```python
from build123d import *

# Parameters (mm, degrees)
SKETCH1_R           = 1.7859375
BOSS_EXTRUDE1_DEPTH = 1.5875
FILLET1_R           = 3.571875


with BuildPart() as part:
    # Sketch1 → Boss-Extrude1 (new body)
    with BuildSketch(Plane.XY):
        with BuildLine():
            ThreePointArc((31.75, -12.7), (35.321875, -9.128125), (31.75, -5.55625))
            ThreePointArc((31.75, -5.55625), (37.30625, 0), (31.75, 5.55625))
            Line((31.75, 5.55625), (25.964019559, 5.55625))
            ThreePointArc((25.964019559, 5.55625), (23.279229109, 11.484009389), (20.594438658, 5.55625))
            Line((20.594438658, 5.55625), (11.155561342, 5.55625))
            ThreePointArc((11.155561342, 5.55625), (8.470770891, 11.484009389), (5.785980441, 5.55625))
            Line((5.785980441, 5.55625), (0, 5.55625))
            ThreePointArc((0, 5.55625), (-5.55625, 0), (0, -5.55625))
            ThreePointArc((0, -5.55625), (-3.571875, -9.128125), (0, -12.7))
            ThreePointArc((0, -12.7), (8.980256121, -8.980256121), (12.7, 0))
            Line((12.7, 0), (19.05, 0))
            ThreePointArc((19.05, 0), (22.769743879, -8.980256121), (31.75, -12.7))
        make_face()
        with BuildLine():
            ThreePointArc((0, -10.9140625), (-1.7859375, -9.128125), (0, -7.3421875))
            ThreePointArc((0, -7.3421875), (5.413228446, -4.960309977), (7.31424826, 0.639913805))
            ThreePointArc((7.31424826, 0.639913805), (8.937735019, 2.574709983), (10.872531197, 0.951223224))
            ThreePointArc((10.872531197, 0.951223224), (8.046690934, -7.37343375), (0, -10.9140625))
        make_face(mode=Mode.SUBTRACT)
        with BuildLine():
            ThreePointArc((24.43575174, 0.639913805), (26.336771554, -4.960309977), (31.75, -7.3421875))
            ThreePointArc((31.75, -7.3421875), (33.5359375, -9.128125), (31.75, -10.9140625))
            ThreePointArc((31.75, -10.9140625), (23.703309066, -7.37343375), (20.877468803, 0.951223224))
            ThreePointArc((20.877468803, 0.951223224), (22.812264981, 2.574709983), (24.43575174, 0.639913805))
        make_face(mode=Mode.SUBTRACT)
        Circle(SKETCH1_R, mode=Mode.SUBTRACT)
        with Locations((8.470770891, 7.912134389)):
            Circle(SKETCH1_R, mode=Mode.SUBTRACT)
        with Locations((31.75, 0)):
            Circle(SKETCH1_R, mode=Mode.SUBTRACT)
        with Locations((23.279229109, 7.912134389)):
            Circle(SKETCH1_R, mode=Mode.SUBTRACT)
    extrude(amount=BOSS_EXTRUDE1_DEPTH)

    # Fillet1
    fillet1_edges = [part.edges().sort_by_distance(p)[0] for p in [
        (31.75, -5.55625, 0.79375),
        (19.05, 0, 0.79375),
        (12.7, 0, 0.79375),
        (0, -5.55625, 0.79375),
        (20.594438658, 5.55625, 0.79375),
        (25.964019559, 5.55625, 0.79375),
        (5.785980441, 5.55625, 0.79375),
        (11.155561342, 5.55625, 0.79375),
    ]]
    fillet(fillet1_edges, radius=FILLET1_R - 0.0001)  # a hair under: the kernel refuses the full size


solid = part.part
```
Source: CAD feature listing. Evaluate the final solid. Frame: model axes, mm. A direction names the side the tool comes from. Coordinates: 2 decimals unless noted, no trailing zeros. Loops run counter-clockwise (first coordinate to the right, second up) from the corner with the lowest first, then second, coordinate; pieces in that order, holes last. Notation, with made-up numbers: M 8.5,-10 L 43.5,-10 A25 ccw 43.5,17 Z; hole C 30,-10 d9. An arc over 180 degrees is marked long. Put each result on its own line as item: value. Start each with the question number.
1) Ray query, L1, parallel to Y at x = 31.75, z = 0.3; L2, parallel to X at y = -4.5, z = 0.35; L3, parallel to X at y = -6.5, z = 0.3. Return the intervals inside material, ascending. Write a range as from..to.
2) Contact query for flat-ended pins moving along their axis: pin 1 Ø3 at (x, y) = (31.75, 0) entering from -Z; pin 2 Ø4 at (x, y) = (8.47, 7.91) entering from -Z. Output: stop coordinate, or through.
3) Cut plane A-A on y = -10.5. Return the cut outline in (x, z), then the cut area to 3 significant figures.
4) Cut plane D-D on z = 0.8. Give the number of separate pieces and of enclosed holes in the cut face, then the cut area to 3 significant figures.
5) Pull-direction query (Y, two-part tool) for faces 1 (the face through (16, 2, 0)), 2 (the face through (8.541, 11.483, 0.783)), 3 (the face through (23.789, -7.466, 0.783)), 4 (the face through (23.72, -9.84, 0.78)); classes: pulls with the +Y half, pulls with the -Y half, needs draft (parallel to the pull), parting line crosses it, or undercut.
6) Cut plane C-C on x = 24. Return the cut outline in (y, z), then the cut area to 3 significant figures.
7) Cut plane B-B on x = 6. Return the cut outline in (y, z), then the cut area to 3 significant figures.
8) Reachability of faces 5 (the face through (22.773, 2.578, 0.783)), 6 (the face through (18.13, -0.8, 0.8)), 7 (the face through (31, 5.556, 1)), 8 (the face through (13.24, 6.37, 0.8)), 9 (the face through (1, 5.556, 1)) from +Z, -Z, +X, -X, +Y, -Y: full face, straight path, thin tool, end or side. Return the list, or none.
The answers:
1. L1: y = -12.7..-10.91, -7.34..-1.79, 1.79..5.56
1. L2: x = -3.51..5.8, 9.94..11.88, 19.87..21.81, 25.95..35.26
1. L3: x = -3.01..3.41, 8.77..10.91, 20.84..22.98, 28.34..34.76
2. pin 1: passes through
2. pin 2: stops at z = 0
3. outline: M -3.3,0 L -1.14,0 L -1.14,1.59 L -3.3,1.59 Z; M 2.98,0 L 7.14,0 L 7.14,1.59 L 2.98,1.59 Z; M 24.61,0 L 28.77,0 L 28.77,1.59 L 24.61,1.59 Z; M 32.89,0 L 35.05,0 L 35.05,1.59 L 32.89,1.59 Z
3. area: 20.1 mm²
4. separate pieces: 1
4. enclosed holes: 6
4. area: 491 mm²
5. face 1: needs draft
5. face 2: pulls with the +Y half
5. face 3: undercut
5. face 4: pulls with the -Y half
6. outline: M -10.06,0 L -7.68,0 L -7.68,1.59 L -10.06,1.59 Z; M 1.97,0 L 6.28,0 L 6.28,1.59 L 1.97,1.59 Z; M 9.55,0 L 11.41,0 L 11.41,1.59 L 9.55,1.59 Z
6. area: 13.6 mm²
7. outline: M -11.19,0 L -9.12,0 L -9.12,1.59 L -11.19,1.59 Z; M -4.23,0 L 10.49,0 L 10.49,1.59 L -4.23,1.59 Z
7. area: 26.7 mm²
8. face 5: +Z, -Z
8. face 6: +Z, -Z, -Y
8. face 7: +Z, -Z, +X, +Y
8. face 8: +Z, -Z, +Y
8. face 9: +Z, -Z, -X, +Y
